```python
from build123d import *

# Parameters (mm, degrees)
F3_D = 36.11626


# Not quite as in the source:
# - a fillet or chamfer that OpenCascade refuses, or shapes differently, is made with other operations: its cross-section is extruded or revolved along the edge and cut away or added


with BuildPart() as f1:
    # F0 (on Front) → F1 (revolve)
    with BuildSketch(Plane.XZ):
        Polygon((0, 0), (0, 34.925), (-104.5604041832, 57.15), (-104.5604041832, 66.675), (-120.65, 66.675), (-120.65, 20.32), (-55.88, 20.32), (-55.88, 0), align=None)
    revolve(axis=Axis((-55.6578852736, 0, 0), (-1, 0, 0)))

    # F3 (through all)
    with Locations(Plane.YZ):
        with Locations((0, 0)):
            Hole(F3_D / 2)

    # F4: chamfer of 1.27 on 5 edges, made by hand

    # F4_s1 → F4_t2 (revolve, cut)
    with BuildSketch(Plane.XZ):
        Polygon((-120.65, 65.405), (-119.38, 66.675), (-120.65, 66.675), align=None)
    revolve(axis=Axis((-120.65, 0, 0), (-1, 0, 0)), mode=Mode.SUBTRACT)

    # F4_s3 → F4_t4 (revolve, cut)
    with BuildSketch(Plane.XZ):
        Polygon((-119.38, 20.32), (-120.65, 21.59), (-120.65, 20.32), align=None)
    revolve(axis=Axis((-120.65, 0, 0), (-1, 0, 0)), mode=Mode.SUBTRACT)

    # F4_s5 → F4_t6 (revolve, cut)
    with BuildSketch(Plane.XZ):
        Polygon((-105.8304041832, 66.675), (-104.5604041832, 65.405), (-104.5604041832, 66.675), align=None)
    revolve(axis=Axis((-104.5604041832, 0, 0), (-1, 0, 0)), mode=Mode.SUBTRACT)

    # F4_s7 → F4_t8 (revolve, cut)
    with BuildSketch(Plane.XZ):
        Polygon((0, 33.8965742778), (-1.0059521527, 35.1388217308), (0, 34.925), align=None)
    revolve(axis=Axis((0, 0, 0), (-1, 0, 0)), mode=Mode.SUBTRACT)

    # F4_s9 → F4_t10 (revolve, cut)
    with BuildSketch(Plane.XY):
        Polygon((-1.27, 18.05813), (0, 19.32813), (0, 18.05813), align=None)
    revolve(axis=Axis((0, 0, 0), (1, 0, 0)), mode=Mode.SUBTRACT)


solid = f1.part
```
Check sheet for the modelled part. Datum: model origin and axes. Units: mm. A direction names the side the tool comes from. Coordinates: 2 decimals unless noted, no trailing zeros. Order: outer loops, then holes, each group sorted by start corner. A loop starts at its lowest first (then second) coordinate and runs counter-clockwise, first axis right, second up. Notation, with made-up numbers: (30, -15.75) -> (51, -15.75) arc R11 cw to (51, -11.75) -> close; hole circle Ø7 at (58.5, 14). An arc over 180 degrees is marked (long way). Write item = value, one per line. Start each with the question number.
1) Go/stop test with flat-tipped pins: P1, Ø1, axis at x = -82.5, z = -14, coming from the +Y side; P2, Ø1.5, axis at x = -86, z = 38.5, coming from the -Y side; P3, Ø3, axis at y = -50.5, z = 43.5, coming from the +X side; P4, Ø12, axis at y = -7, z = -2, coming from the -X side. Record where each tip stops, or that it passes through.
2) Access from +Z, -Z, +X, -X, +Y, -Y to the whole of each face (thin tool, end or side, straight path). Record for faces 1 (the flat face through (-104.56, -58, 0)), 2 (the flat face through (-55.88, 18.2, -1.6)), 3 (the flat face through (0, -15, -15)).
3) Cross-section at C-C (x = -16.5). Enter the section's corners in (y, z), then the cut area to 3 significant figures.
4) Cross-section at A-A (y = 0). Enter the section's corners in (x, z) (3 decimals), then the cut area to 3 significant figures.
5) Mould release check, pull along Y, two halves, no side actions. Record for faces 4 (the cylindrical face through (-28.96, 3.91, -17.63)), 5 (the cylindrical face through (-87.185, 20.147, -2.645)), 6 (the cylindrical face through (-112.7, 20.027, 63.596)), 7 (the flat face through (-120.65, 15.5, -15.5)): +Y half, -Y half, draft (parallel to the pull), parting line (faces both ways), or undercut.
6) Material ranges on L1, parallel to X at y = -13.5, z = 61.5; L2, parallel to Y at x = -96, z = 5; L3, parallel to Z at x = -34, y = 0, recorded low to high.
7) Cross-section at D-D (x = -73.5). Enter the section's corners in (y, z), then the cut area to 3 significant figures.
Ans:
q1.P1 = 50.73
q1.P2 = -37.53
q1.P3 = -104.56
q1.P4 = through
q2.face_1 = +X
q2.face_2 = -X
q2.face_3 = +Z, -Z, +X, +Y, -Y
q3.outline = circle Ø76.86 at (0, 0); hole circle Ø36.12 at (0, 0)
q3.area = 3,620 mm²
q4.outline = (-120.65, -65.405) -> (-119.38, -66.675) -> (-105.83, -66.675) -> (-104.56, -65.405) -> (-104.56, -57.15) -> (-1.006, -35.139) -> (0, -33.897) -> (0, -19.328) -> (-1.27, -18.058) -> (-55.88, -18.058) -> (-55.88, -20.32) -> (-119.38, -20.32) -> (-120.65, -21.59) -> close; (-120.65, 21.59) -> (-119.38, 20.32) -> (-55.88, 20.32) -> (-55.88, 18.058) -> (-1.27, 18.058) -> (0, 19.328) -> (0, 33.897) -> (-1.006, 35.139) -> (-104.56, 57.15) -> (-104.56, 65.405) -> (-105.83, 66.675) -> (-119.38, 66.675) -> (-120.65, 65.405) -> close
q4.area = 7,120 mm²
q5.face_4 = undercut
q5.face_5 = undercut
q5.face_6 = parting line
q5.face_7 = draft
q6.L1 = -120.65 to -104.56
q6.L2 = -55.1 to -19.7, 19.7 to 55.1
q6.L3 = -42.15 to -18.06, 18.06 to 42.15
q7.outline = circle Ø101.1 at (0, 0); hole circle Ø40.64 at (0, 0)
q7.area = 6,730 mm²
